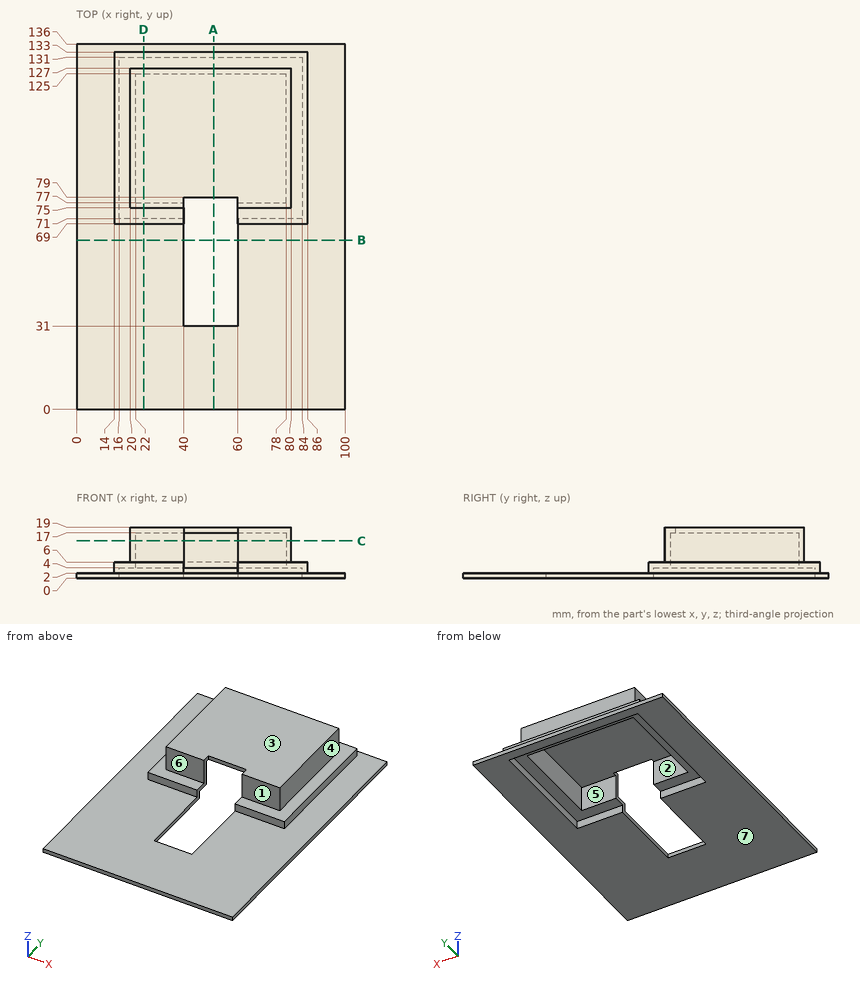
Could you check a few things on this drawing? It's one solid part, dimensions in mm from its lowest x, y, z. A direction names the side the tool comes from. Round coordinates to 2 decimals unless told otherwise and drop trailing zeros. Write each loop counter-clockwise with the first axis right and the second up, starting at its lowest first coordinate (ties: lowest second). Pieces come first, ordered by that corner, then holes.
Q1. Please list where these lines run through material, in increasing order: probe 1 along Y at (x, z) = (24, 10); probe 2 along X at (y, z) = (130, 3.25); probe 3 along Y at (x, z) = (24, 2.5).
Q2. If we section it at B-B on y = 63: Write out the boundary of the cut face in (x, z).
Q3. If we section it at C-C on z = 14: Write out the boundary of the cut face in (x, y).
Q4. Will these pins go through, and if not, where does the flat tip stop? P1, Ø1, axis at x = 12, y = 68, coming from the +Z side; P2, Ø1.2, axis at x = 49.5, z = 4, coming from the +Y side; P3, Ø10, axis at x = 83, z = 9.5, coming from the -Y side; P4, Ø1.2, axis at x = 53.5, z = 2.5, coming from the -Y side.
Q5. If we section it at A-A on x = 51: Write out the boundary of the cut face in (y, z), plus the area to 3 significant figures.
Q6. Which directions (+Z, -Z, +X, -X, +Y, -Y) give clear straight access to the entire face, cutting with the end or side of a thin tool? Please do the marked faces 1, 2, 3 and 4.
Q7. If we section it at D-D on x = 25: Write out the boundary of the cut face in (y, z), plus the area to 3 significant figures.
Q8. If we mould it in two halves opening along Y, with no side actions, what happens to the marked faces 5, 6 and 7? For each: +Y half, -Y half, draft (parallel to the pull), parting line (faces both ways), or undercut.
Answer below:
1. probe 1: y = 75 to 77, 125 to 127
1. probe 2: x = 14 to 16, 84 to 86
1. probe 3: y = 69 to 71, 131 to 133
2. outline: (0, 0) - (40, 0) - (40, 2) - (0, 2) - close; (60, 0) - (100, 0) - (100, 2) - (60, 2) - close
3. outline: (20, 75) - (40, 75) - (40, 77) - (22, 77) - (22, 125) - (78, 125) - (78, 77) - (60, 77) - (60, 75) - (80, 75) - (80, 127) - (20, 127) - close
4. P1: stops at z = 2
4. P2: stops at y = 133
4. P3: stops at y = 69
4. P4: stops at y = 0
5. outline: (0, 0) - (31, 0) - (31, 2) - (0, 2) - close; (79, 17) - (125, 17) - (125, 4) - (131, 4) - (131, 0) - (136, 0) - (136, 2) - (133, 2) - (133, 6) - (127, 6) - (127, 19) - (79, 19) - close
5. area: 210 mm2
6. face 1: +Z, +X, -X, -Y
6. face 2: -Z
6. face 3: +Z, +X, -X, +Y, -Y
6. face 4: +Z, +X, +Y, -Y
7. outline: (0, 0) - (71, 0) - (71, 4) - (77, 4) - (77, 17) - (125, 17) - (125, 4) - (131, 4) - (131, 0) - (136, 0) - (136, 2) - (133, 2) - (133, 6) - (127, 6) - (127, 19) - (75, 19) - (75, 6) - (69, 6) - (69, 2) - (0, 2) - close
7. area: 340 mm2
8. face 5: undercut
8. face 6: -Y half
8. face 7: draft
